Here's how the part is built. I have some questions about the finished solid (model axes, mm). A direction names the side the tool comes from. Give positions to 0.01 mm unless a question says otherwise; leave off trailing zeros. Write each loop counter-clockwise with the first axis right and the second up, starting at its lowest first coordinate (ties: lowest second). Pieces come first, ordered by that corner, then holes. Notation, with made-up numbers: (55.25, 86) - (92.25, 86) arc R24 ccw to (92.25, 107) - close; hole circle Ø4 at (2.5, -23.75). An arc over 180 degrees is marked (long way). Use a Markdown table: item, result.
```python
from build123d import *

# Parameters (mm, degrees)
SKETCH_1_W          = 42
SKETCH_1_H          = 42
EXTRUDE_1_DEPTH     = 5
SKETCH_3_R          = 11
SKETCH_3_R_2        = 1.5
CUT_EXTRUDE_1_DEPTH = 31.116440693
SKETCH_2_R          = 1.5
CUT_EXTRUDE_3_DEPTH = 4


with BuildPart() as part:
    # 스케치1 → 보스-돌출1 (new body)
    with BuildSketch(Plane(origin=(0, 0, 0), x_dir=(1, 0, 0), z_dir=(0, 1, 0))):
        Rectangle(SKETCH_1_W, SKETCH_1_H)
    extrude(amount=EXTRUDE_1_DEPTH)

    # 스케치3 → 컷-돌출1 (cut, through all)
    with BuildSketch(Plane(origin=(0, 5, 0), x_dir=(1, 0, 0), z_dir=(0, 1, 0))):
        with Locations(Location((0, 0, 0), (0, 0, 270))):
            Circle(SKETCH_3_R)
        with Locations(Location((-15.5, 15.5, 0), (0, 0, 270))):
            Circle(SKETCH_3_R_2)
        with Locations(Location((15.499999997, 15.49956129, 0), (0, 0, 270))):
            Circle(SKETCH_3_R_2)
        with Locations(Location((15.499561287, -15.500438707, 0), (0, 0, 270))):
            Circle(SKETCH_3_R_2)
        with Locations(Location((-15.50043871, -15.499999997, 0), (0, 0, 270))):
            Circle(SKETCH_3_R_2)
    extrude(amount=-CUT_EXTRUDE_1_DEPTH, mode=Mode.SUBTRACT)

    # 스케치2 → 컷-돌출3 (cut)
    with BuildSketch(Plane.XY.offset(21)):
        with Locations((-18.5, 2.5)):
            Circle(SKETCH_2_R)
        with Locations((18.5, 2.5)):
            Circle(SKETCH_2_R)
        with Locations((0, 2.5)):
            Circle(SKETCH_2_R)
    extrude(amount=-CUT_EXTRUDE_3_DEPTH, mode=Mode.SUBTRACT)


solid = part.part
```
Item 1: For faces 1 (the flat face through (-21, 2, 0)), 2 (the flat face through (-19, 3, 17)), which set-ups out of +Z, -Z, +X, -X, +Y, -Y let a thin tool reach every point of the face, with its end or its side?
Values:
| item | result |
|---|---|
| face 1 | +Z, -Z, -X, +Y, -Y |
| face 2 | +Z |
Item 2: Will this pin go through, and if not, where does the flat tip stop? pin 1 Ø1.5 at (x, y) = (19, 2) entering from +Z.
Values:
| item | result |
|---|---|
| pin 1 | stops at z = 17 |
Item 3: If we section it at D-D, the plane x = 18.5: Write out the boundary of the cut face in (y, z), plus the area to 3 significant figures.
Values:
| item | result |
|---|---|
| outline | (0, -21) - (5, -21) - (5, 21) - (4, 21) - (4, 17) - (1, 17) - (1, 21) - (0, 21) - close |
| area | 198 mm2 |
Item 4: If we section it at C-C, the plane z = -5: Write out the boundary of the cut face in (x, y).
Values:
| item | result |
|---|---|
| outline | (-21, 0) - (-9.8, 0) - (-9.8, 5) - (-21, 5) - close; (9.8, 0) - (21, 0) - (21, 5) - (9.8, 5) - close |
Item 5: Thinking about a two-plate mould opening in Z: for faces 3 (the flat face through (-10, 5, -10)), 4 (the cylindrical face through (-15.43, 2.54, -17)), 5 (the flat face through (0, 2, -21)), which applies, +Z half, -Z half, draft (parallel to the pull), parting line (faces both ways), or undercut?
Values:
| item | result |
|---|---|
| face 3 | draft |
| face 4 | undercut |
| face 5 | -Z half |
Item 6: If we section it at A-A, the plane z = 15.5: Write out the boundary of the cut face in (x, y).
Values:
| item | result |
|---|---|
| outline | (-21, 0) - (-17, 0) - (-17, 5) - (-21, 5) - close; (-14, 0) - (14, 0) - (14, 5) - (-14, 5) - close; (17, 0) - (21, 0) - (21, 5) - (17, 5) - close |
Item 7: If we section it at B-B, the plane x = 0: Write out the boundary of the cut face in (y, z), plus the area to 3 significant figures.
Values:
| item | result |
|---|---|
| outline | (0, -21) - (5, -21) - (5, -11) - (0, -11) - close; (0, 11) - (5, 11) - (5, 21) - (4, 21) - (4, 17) - (1, 17) - (1, 21) - (0, 21) - close |
| area | 88.0 mm2 |
Item 8: I need wall thicknesses on line 1 along X through (y, z) = (2.3, 15.5); line 2 along Y through (x, z) = (18.5, 18.55). Which ranges of each line are inside material? Lowest first, please. Write a range as [from, to].
Values:
| item | result |
|---|---|
| line 1 | x = [-21, -17], [-14, 14], [17, 21] |
| line 2 | y = [0, 1], [4, 5] |
